Geometry: final body of the model. Coordinates: model frame, mm. Give positions to 0.01 mm unless a question says otherwise; leave off trailing zeros. Write each loop counter-clockwise with the first axis right and the second up, starting at its lowest first coordinate (ties: lowest second). Pieces come first, ordered by that corner, then holes.
from build123d import *

# Parameters (mm, degrees)
F0_W     = 120
F0_H     = 50
F1_DEPTH = 3
F2_R     = 2.5
F2_R_2   = 5.0292
F3_DEPTH = 3.001


with BuildPart() as f1:
    # F0 (on Front) → F1 (new body)
    with BuildSketch(Plane.XZ):
        Rectangle(F0_W, F0_H)
    extrude(amount=F1_DEPTH)

    # F2 (on face) → F3 (cut, through all)
    with BuildSketch(Plane.XZ.offset(3)):
        with Locations((-50, 0)):
            Circle(F2_R)
        with Locations((-49.6740713716, -19.0056)):
            Circle(F2_R)
        with Locations((-29.8628, 0)):
            Circle(F2_R_2)
        with Locations((-10, 0)):
            Circle(F2_R)
        with Locations((-9.6392054111, -18.9992)):
            Circle(F2_R)
        with Locations((12, 12)):
            Circle(F2_R)
        with Locations((12, -12)):
            Circle(F2_R)
        with Locations((30, 0)):
            Circle(F2_R_2)
        with Locations((30, -18.9992)):
            Circle(F2_R)
        with Locations((52.5, 12)):
            Circle(F2_R)
        with Locations((52.5, -12)):
            Circle(F2_R)
        with BuildLine():
            ThreePointArc((-7.5, 19), (-10, 21.5), (-12.5, 19))
            Line((-12.5, 19), (-7.5, 19))
        make_face()
        with BuildLine():
            Line((-7.5, 19), (-12.5, 19))
            ThreePointArc((-12.5, 19), (-10, 16.5), (-7.5, 19))
        make_face()
        with BuildLine():
            ThreePointArc((32.5, 19), (30, 21.5), (27.5, 19))
            Line((27.5, 19), (32.5, 19))
        make_face()
        with BuildLine():
            Line((32.5, 19), (27.5, 19))
            ThreePointArc((27.5, 19), (30, 16.5), (32.5, 19))
        make_face()
        with Locations((-50, 19)):
            Circle(F2_R)
    extrude(amount=-F3_DEPTH, mode=Mode.SUBTRACT)


solid = f1.part
Q1. Section B-B on x = 30. Output: boundary loops of the cut face in (y, z).
Filled sheet:
outline: (-3, -25) - (0, -25) - (0, -21.5) - (-3, -21.5) - close; (-3, -16.5) - (0, -16.5) - (0, -5.03) - (-3, -5.03) - close; (-3, 5.03) - (0, 5.03) - (0, 16.5) - (-3, 16.5) - close; (-3, 21.5) - (0, 21.5) - (0, 25) - (-3, 25) - close
Q2. Section A-A on z = 19. Output: boundary loops of the cut face in (x, y), plus the area to 3 significant figures.
Filled sheet:
outline: (-60, -3) - (-52.5, -3) - (-52.5, 0) - (-60, 0) - close; (-47.5, -3) - (-12.5, -3) - (-12.5, 0) - (-47.5, 0) - close; (-7.5, -3) - (27.5, -3) - (27.5, 0) - (-7.5, 0) - close; (32.5, -3) - (60, -3) - (60, 0) - (32.5, 0) - close
area: 315 mm2
Q3. Pin query (flat end, axial travel): P1, Ø3, axis at x = 30, z = 19, coming from the -Y side. Return the tip coordinate at first contact, or that it passes through.
Filled sheet:
P1: passes through
Q4. Pull-direction query (X, two-part tool) for faces 1 (the flat face through (60, -1, 0)), 2 (the cylindrical face through (-47.365, -1.521, -19.963)), 3 (the flat face through (-1, -1, 25)); classes: released by +X, released by -X, zero draft, split by the parting line, or undercut.
Filled sheet:
face 1: released by +X
face 2: undercut
face 3: zero draft
Q5. Section C-C on z = 0. Output: boundary loops of the cut face in (x, y).
Filled sheet:
outline: (-60, -3) - (-52.5, -3) - (-52.5, 0) - (-60, 0) - close; (-47.5, -3) - (-34.89, -3) - (-34.89, 0) - (-47.5, 0) - close; (-24.83, -3) - (-12.5, -3) - (-12.5, 0) - (-24.83, 0) - close; (-7.5, -3) - (24.97, -3) - (24.97, 0) - (-7.5, 0) - close; (35.03, -3) - (60, -3) - (60, 0) - (35.03, 0) - close
Q6. Section D-D on x = 52.5. Output: boundary loops of the cut face in (y, z).
Filled sheet:
outline: (-3, -25) - (0, -25) - (0, -14.5) - (-3, -14.5) - close; (-3, -9.5) - (0, -9.5) - (0, 9.5) - (-3, 9.5) - close; (-3, 14.5) - (0, 14.5) - (0, 25) - (-3, 25) - close
Q7. Ray query, line 1 along X through (y, z) = (-1.3, -19); line 2 along Z through (x, y) = (52.5, -1.3); line 3 along Z through (x, y) = (-50, -1.6). Return the intervals inside material, ascending.
Filled sheet:
line 1: x = -60 to -52.17, -47.17 to -12.14, -7.14 to 27.5, 32.5 to 60
line 2: z = -25 to -14.5, -9.5 to 9.5, 14.5 to 25
line 3: z = -25 to -21.48, -16.53 to -2.5, 2.5 to 16.5, 21.5 to 25
